Autodesk Inventor part; units mm, degrees
ref_plane "YZ Plane" through (0, 0, 0) normal (1, 0, 0) x (0, 1, 0)
ref_plane "XZ Plane" through (0, 0, 0) normal (0, 1, 0) x (-1, 0, 0)
ref_plane "XY Plane" through (0, 0, 0) normal (0, 0, 1) x (1, 0, 0)
sketch "Sketch1" plane through (0, 0, 0) normal (0, 0, 1) x (1, 0, 0)
  line L0 (-17.78, 0) -> (17.78, 0)
  line L1 (0, -17.78) -> (0, 17.78)
  line L2 (-12.7, 12.7) -> (12.7, 12.7)
  line L3 (12.7, 12.7) -> (12.7, -12.7)
  line L4 (12.7, -12.7) -> (-12.7, -12.7)
  line L5 (-12.7, -12.7) -> (-12.7, 12.7)
  line L6 (9.525, 9.525) -> (-9.525, 9.525)
  line L7 (-9.525, 9.525) -> (-9.525, -9.525)
  line L8 (-9.525, -9.525) -> (9.525, -9.525)
  line L9 (9.525, -9.525) -> (9.525, 9.525)
  point P0 (0, 0)
  point P1 (-12.7, 0)
  point P2 (0, 12.7)
  dimension "d0" = 25.4
  dimension "d1" = 3.175
extrude "Base" add sketch "Sketch1" along normal mid plane 322.2625 contours L5 L2 L1 L6 L7 L0 | L0 L7 L8 L1 L4 L5 | L1 L8 L9 L0 L3 L4 | L2 L3 L0 L9 L6 L1
sketch "Sketch6" plane through (-12.7, 12.7, 161.1312) normal (0, 1, 0) x (1, 0, 0)
  line L0 (0, 0) -> (25.4, 0)
  line L1 (0, 322.2625) -> (0, 0)
  line L2 (25.4, 0) -> (0, 14.6647)
  point P0 (12.7, 161.1312)
  dimension "d15" = 30
extrude "Extrusion6" cut sketch "Sketch6" against normal through all
sketch "Sketch7" plane through (-12.7, 12.7, -161.1312) normal (0, 1, 0) x (1, 0, 0)
  line L0 (25.4, 0) -> (0, 0)
  line L1 (0, 0) -> (0, -307.5978)
  line L2 (25.4, 0) -> (0, -14.6647)
  point P0 (12.7, -161.1312)
  dimension "d18" = 30
extrude "Extrusion7" cut sketch "Sketch7" against normal through all
properties part number "tubing_template_0.125" material "Aluminum-6061"
Here's how the part is built. I have some questions about the finished solid (model axes, mm). A direction names the side the tool comes from. Round coordinates to 2 decimals unless told otherwise and drop trailing zeros. Order: outer loops, then holes, each group sorted by start corner. A loop starts at its lowest first (then second) coordinate and runs counter-clockwise, first axis right, second up. Notation, with made-up numbers: (20, 10.5) -> (48, 10.5) arc R25 ccw to (48, 33.5) -> close; hole circle Ø7 at (22.25, 58.5). An arc over 180 degrees is marked (long way). Use CSV: the item, a comma, the result in double quotes.
1. I need wall thicknesses on line 1 along X through (y, z) = (-4.25, 63) (3 decimals); line 2 along Z through (x, y) = (9, -11) (3 decimals). Which ranges of each line are inside material? Lowest first, please.
Recorded:
line 1,"x = -12.7 to -9.525, 9.525 to 12.7"
line 2,"z = -158.995 to 158.995"
2. I want a section at A-A on z = 30. List the corners of the cut face in (x, y) for me (3 decimals), and give its area (3 significant figures).
Recorded:
outline,"(-12.7, -12.7) -> (12.7, -12.7) -> (12.7, 12.7) -> (-12.7, 12.7) -> close; hole (-9.525, -9.525) -> (9.525, -9.525) -> (9.525, 9.525) -> (-9.525, 9.525) -> close"
area,"282 mm2"
3. I want a section at C-C on y = -1.5. List the corners of the cut face in (x, z) for me (1 decimal), and give its area (3 significant figures).
Recorded:
outline,"(-12.7, -146.5) -> (-9.5, -148.3) -> (-9.5, 148.3) -> (-12.7, 146.5) -> close; (9.5, -159.3) -> (12.7, -161.1) -> (12.7, 161.1) -> (9.5, 159.3) -> close"
area,"1,950 mm2"
4. Thinking about a two-plate mould opening in Y: for faces 3 (the face through (12.7, 0, -2)), 4 (the face through (0, 9.525, -2)), 5 (the face through (0, -12.7, -2)), 6 (the face through (9.525, 0, -2)), which applies, pulls with the +Y half, pulls with the -Y half, needs draft (parallel to the pull), parting line crosses it, or undercut?
Recorded:
face 3,"needs draft"
face 4,"undercut"
face 5,"pulls with the -Y half"
face 6,"undercut"
5. I want a section at B-B on x = 0. List the corners of the cut face in (y, z) for me (3 decimals).
Recorded:
outline,"(-12.7, -153.799) -> (-9.525, -153.799) -> (-9.525, 153.799) -> (-12.7, 153.799) -> close; (9.525, -153.799) -> (12.7, -153.799) -> (12.7, 153.799) -> (9.525, 153.799) -> close"
6. Which directions (+Z, -Z, +X, -X, +Y, -Y) give clear straight access to the entire face, cutting with the end or side of a thin tool? Please do faces 1 (the face through (0.178, -11.111, 153.902)), 2 (the face through (0, -9.525, -2)).
Recorded:
face 1,"+Z, -X, +Y, -Y"
face 2,"+Z, -Z"
